```python
from build123d import *

# Parameters (mm, degrees)
SKETCH1_W           = 64.008
SKETCH1_H           = 68.834
BOSS_EXTRUDE1_DEPTH = 3.048
SKETCH2_W           = 3.048
SKETCH2_H           = 68.834
BOSS_EXTRUDE2_DEPTH = 6.858
SKETCH3_W           = 1.016
SKETCH3_H           = 1.905
CUT_EXTRUDE1_DEPTH  = 95.515990478
SKETCH4_W           = 3.048
SKETCH4_H           = 68.834
BOSS_EXTRUDE3_DEPTH = 6.858
SKETCH5_W           = 1.016
SKETCH5_H           = 1.905
CUT_EXTRUDE2_DEPTH  = 95.515990478


with BuildPart() as part:
    # Sketch1 → Boss-Extrude1 (new body)
    with BuildSketch(Plane(origin=(0, 0, 0), x_dir=(1, 0, 0), z_dir=(0, 1, 0))):
        with Locations((32.004, 34.417)):
            Rectangle(SKETCH1_W, SKETCH1_H)
    extrude(amount=BOSS_EXTRUDE1_DEPTH)

    # Sketch2 → Boss-Extrude2 (add)
    with BuildSketch(Plane(origin=(0, 3.048, 0), x_dir=(1, 0, 0), z_dir=(0, 1, 0))):
        with Locations((58.166, 34.417)):
            Rectangle(SKETCH2_W, SKETCH2_H)
    extrude(amount=BOSS_EXTRUDE2_DEPTH)

    # Sketch3 → Cut-Extrude1 (cut, through all)
    with BuildSketch(Plane.XY):
        with Locations((57.15, 5.9055)):
            Rectangle(SKETCH3_W, SKETCH3_H)
    extrude(amount=-CUT_EXTRUDE1_DEPTH, mode=Mode.SUBTRACT)

    # Sketch4 → Boss-Extrude3 (add)
    with BuildSketch(Plane(origin=(0, 3.048, 0), x_dir=(1, 0, 0), z_dir=(0, 1, 0))):
        with Locations((3.302, 34.417)):
            Rectangle(SKETCH4_W, SKETCH4_H)
    extrude(amount=BOSS_EXTRUDE3_DEPTH)

    # Sketch5 → Cut-Extrude2 (cut, through all)
    with BuildSketch(Plane.XY):
        with Locations((4.318, 5.9055)):
            Rectangle(SKETCH5_W, SKETCH5_H)
    extrude(amount=-CUT_EXTRUDE2_DEPTH, mode=Mode.SUBTRACT)


solid = part.part
```
Check sheet for the modelled part. Datum: model origin and axes. Units: mm. A direction names the side the tool comes from. Coordinates: 2 decimals unless noted, no trailing zeros. Loops run counter-clockwise (first coordinate to the right, second up) from the corner with the lowest first, then second, coordinate; pieces in that order, holes last.
1) Sectioned sample at C-C (x = 38). Record the boundary of the cut face in (y, z).
2) Material ranges on probe 1 along X at (y, z) = (6, -22.5); probe 2 along Y at (x, z) = (57, -7.5); probe 3 along X at (y, z) = (8.5, -21.5), recorded low to high.
3) Access from +Z, -Z, +X, -X, +Y, -Y to the whole of each face (thin tool, end or side, straight path). Record for faces 1 (the face through (1, 3.048, -35)), 2 (the face through (62, 3.048, -35)), 3 (the face through (3.81, 6, -34)), 4 (the face through (30, 3.048, -35)).
4) Sectioned sample at B-B (z = -47). Record the boundary of the cut face in (x, y), and give its area (3 significant figures).
5) Release check for a two-part mould opening along Y. For faces 5 (the face through (57.658, 6, -34)), 6 (the face through (32, 0, -35)), 7 (the face through (1.778, 6, -34)) record: released by +Y, released by -Y, zero draft, split by the parting line, or undercut.
6) Gauge pin test, flat ends, axial feed: pin 1 (0.6 mm diameter, centred on y = 4, z = -22, fed in from -X); pin 2 (1.3 mm diameter, centred on x = 62, z = -31.5, fed in from +Y); pin 3 (0.6 mm diameter, centred on y = 3.5, z = -46, fed in from +X); pin 4 (4 mm diameter, centred on x = 44.5, y = 6, fed in from +Z). Record the tip position at first contact, or that the pin passes through.
7) Sectioned sample at A-A (y = 5.75). Record the boundary of the cut face in (x, z).
Check sheet entries:
1. outline: (0, -68.83) - (3.05, -68.83) - (3.05, 0) - (0, 0) - close
2. probe 1: x = 1.78 to 3.81, 57.66 to 59.69
2. probe 2: y = 0 to 4.95, 6.86 to 9.91
2. probe 3: x = 1.78 to 4.83, 56.64 to 59.69
3. face 1: +Z, -Z, -X, +Y
3. face 2: +Z, -Z, +X, +Y
3. face 3: +Z, -Z
3. face 4: +Z, -Z, +Y
4. outline: (0, 0) - (64.01, 0) - (64.01, 3.05) - (59.69, 3.05) - (59.69, 9.91) - (56.64, 9.91) - (56.64, 6.86) - (57.66, 6.86) - (57.66, 4.95) - (56.64, 4.95) - (56.64, 3.05) - (4.83, 3.05) - (4.83, 4.95) - (3.81, 4.95) - (3.81, 6.86) - (4.83, 6.86) - (4.83, 9.91) - (1.78, 9.91) - (1.78, 3.05) - (0, 3.05) - close
4. area: 233 mm2
5. face 5: undercut
5. face 6: released by -Y
5. face 7: zero draft
6. pin 1: stops at x = 1.78
6. pin 2: stops at y = 3.05
6. pin 3: stops at x = 59.69
6. pin 4: passes through
7. outline: (1.78, -68.83) - (3.81, -68.83) - (3.81, 0) - (1.78, 0) - close; (57.66, -68.83) - (59.69, -68.83) - (59.69, 0) - (57.66, 0) - close
